Autodesk Inventor part; units mm, degrees
ref_plane "YZ Plane" through (0, 0, 0) normal (1, 0, 0) x (0, 1, 0)
ref_plane "XZ Plane" through (0, 0, 0) normal (0, 1, 0) x (-1, 0, 0)
ref_plane "XY Plane" through (0, 0, 0) normal (0, 0, 1) x (1, 0, 0)
sketch "Sketch1" plane through (0, 0, 0) normal (0, 0, 1) x (1, 0, 0)
  circle A0 centre (0, 0) radius 17.7488
extrude "Extrusion1" add sketch "Sketch1" along normal blind 21.45
sketch "Sketch2" plane through (0, 0, 0) normal (0, 0, -1) x (-1, 0, 0)
  circle A0 centre (0, 0) radius 16.574
extrude "Extrusion2" add sketch "Sketch2" along normal blind 18.2
sketch "Sketch5" plane through (0, 0, 21.45) normal (0, 0, 1) x (1, 0, 0)
  circle A0 centre (0, 0) radius 18.1003
extrude "Extrusion5" add sketch "Sketch5" along normal blind 1
sketch "Sketch3" plane through (0, 0, -18.2) normal (0, 0, -1) x (-1, 0, 0)
  circle A0 centre (0, 0) radius 17.7488
  line L0 (17.7488, 0) -> (14.2875, 0)
  circle A1 centre (0, 0) radius 16.574
  line L1 (15.3093, 6.35) -> (15.3093, -6.35)
  circle A2 centre (3.175, 7.9375) radius 1.5875
extrude "Extrusion3" add sketch "Sketch3" against normal blind 10 contours A2
sketch "Sketch4" plane through (0, 0, -18.2) normal (0, 0, -1) x (-1, 0, 0)
  circle A0 centre (3.175, -4.7625) radius 1.5875
  point P0 (0, 0)
extrude "Extrusion4" cut sketch "Sketch4" against normal blind 10
sketch "Sketch6" plane through (0, 0, 22.45) normal (0, 0, 1) x (1, 0, 0)
  point P0 (0, 0)
sketch "Sketch7" plane through (0, 0, 22.45) normal (0, 0, 1) x (1, 0, 0)
  line L0 (7.9375, 4.7625) -> (8.0932, -4.4928)
  line L1 (8.0932, -4.4928) -> (0.1557, -9.2553)
  line L2 (0.1557, -9.2553) -> (-7.9375, -4.7625)
  line L3 (-7.9375, -4.7625) -> (-8.0932, 4.4928)
  line L4 (-8.0932, 4.4928) -> (-0.1557, 9.2553)
  line L5 (-0.1557, 9.2553) -> (7.9375, 4.7625)
  point P0 (0, 0)
  point P1 (0, 0)
sketch "Sketch8" plane through (0, 0, 22.45) normal (0, 0, 1) x (1, 0, 0)
  point P0 (0, 0)
extrude "Extrusion6" add sketch "Sketch7" along normal blind 7
sketch "Sketch9" plane through (0, 0, 29.45) normal (0, 0, 1) x (1, 0, 0)
  circle A0 centre (0, 0) radius 3.175
extrude "Extrusion7" add sketch "Sketch9" along normal blind 20
properties part number "DC MOTOR1" material "Iron, Gray"
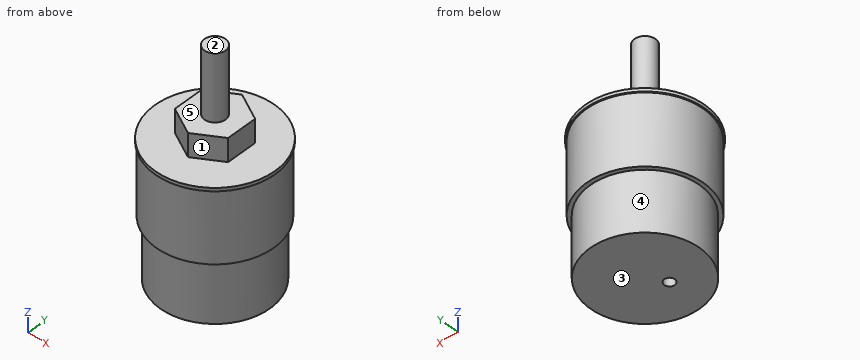
CAD build for the part. Positions are in the model's coordinates, mm. Face numbers are marked on the shaded views. A direction names the side the tool comes from. Round coordinates to 2 decimals unless told otherwise and drop trailing zeros. Loops run counter-clockwise (first coordinate to the right, second up) from the corner with the lowest first, then second, coordinate; pieces in that order, holes last.
(1) Cut at C-C (y = -13). Give the cut face in (x, z), plus the area to 3 significant figures.
(2) Wall check: line 1 along Z through (x, y) = (-12.5, -5); line 2 along Y through (x, z) = (-0.5, 3.5); line 3 along Z through (x, y) = (-4, -3). Give the ranges that are in metal, low to high.
(3) Cut at A-A (x = -10). Give the cut face in (y, z).
(4) Cut at B-B (z = 43). Give the cut face in (x, y) (3 decimals).
(5) Cut at D-D (y = 0). Give the cut face in (x, z) (3 decimals), plus the area to 3 significant figures.
(6) Which spindle directions (+Z, -Z, +X, -X, +Y, -Y) get a long thin tool onto all of the face, cutting with end or side? Do the marked faces 1, 2, 3, 4 and 5. Say none if no direction does.
(7) Drop flat-ended pins along their axis: pin 1 (8 mm diameter, centred on x = -1.5, z = 21.5, fed in from +Y); pin 2 (2 mm diameter, centred on x = 13, z = -2.5, fed in from +Y); pin 3 (8 mm diameter, centred on x = -3, z = 15, fed in from -Y). Give the stop position or say it passes through.
Findings below:
1. outline: (-12.59, 21.45) - (-12.08, 21.45) - (-12.08, 0) - (-10.28, 0) - (-10.28, -18.2) - (10.28, -18.2) - (10.28, 0) - (12.08, 0) - (12.08, 21.45) - (12.59, 21.45) - (12.59, 22.45) - (-12.59, 22.45) - close
1. area: 918 mm2
2. line 1: z = -18.2 to 22.45
2. line 2: y = -17.74 to 17.74
2. line 3: z = -18.2 to 29.45
3. outline: (-15.09, 21.45) - (-14.66, 21.45) - (-14.66, 0) - (-13.22, 0) - (-13.22, -18.2) - (13.22, -18.2) - (13.22, 0) - (14.66, 0) - (14.66, 21.45) - (15.09, 21.45) - (15.09, 22.45) - (-15.09, 22.45) - close
4. outline: circle Ø6.35 at (0, 0)
5. outline: (-18.1, 21.45) - (-17.749, 21.45) - (-17.749, 0) - (-16.574, 0) - (-16.574, -18.2) - (16.574, -18.2) - (16.574, 0) - (17.749, 0) - (17.749, 21.45) - (18.1, 21.45) - (18.1, 22.45) - (8.018, 22.45) - (8.018, 29.45) - (3.175, 29.45) - (3.175, 49.45) - (-3.175, 49.45) - (-3.175, 29.45) - (-8.018, 29.45) - (-8.018, 22.45) - (-18.1, 22.45) - close
5. area: 1,640 mm2
6. face 1: +Z, +X, -Y
6. face 2: +Z, +X, -X, +Y, -Y
6. face 3: -Z, +X, -X, +Y, -Y
6. face 4: -Z
6. face 5: +Z
7. pin 1: stops at y = 18.1
7. pin 2: stops at y = 11.43
7. pin 3: stops at y = -17.75
